CAD build for the part. Positions are in the model's coordinates, mm. A direction names the side the tool comes from. Give positions to 0.01 mm unless a question says otherwise; leave off trailing zeros. Order: outer loops, then holes, each group sorted by start corner. A loop starts at its lowest first (then second) coordinate and runs counter-clockwise, first axis right, second up.
from build123d import *

# Parameters (mm, degrees)
F0_R     = 16.5
F1_DEPTH = 30
F2_W     = 12.5
F2_H     = 30
F3_DEPTH = 17
F4_R     = 9.5
F5_DEPTH = 15
F6_R     = 10.5
F7_DEPTH = 15
F8_R     = 5
F9_DEPTH = 77


with BuildPart() as f1:
    # F0 (on Front) → F1 (new body)
    with BuildSketch(Plane.XZ):
        Circle(F0_R)
    extrude(amount=F1_DEPTH)

    # F2 (on Top) → F3 (join)
    with BuildSketch(Plane.XY):
        with Locations((6.25, -15)):
            Rectangle(F2_W, F2_H)
        with Locations((-6.25, -15)):
            Rectangle(F2_W, F2_H)
    extrude(amount=F3_DEPTH)

    # F4 (on face) → F5 (join)
    with BuildSketch(Plane.XZ.offset(30)):
        Circle(F4_R)
    extrude(amount=F5_DEPTH)

    # F6 (on Front) → F7 (cut)
    with BuildSketch(Plane.XZ):
        Circle(F6_R)
    extrude(amount=F7_DEPTH, mode=Mode.SUBTRACT)

    # F8 (on face) → F9 (cut)
    with BuildSketch(Plane.XZ.offset(45)):
        Circle(F8_R)
    extrude(amount=-F9_DEPTH, mode=Mode.SUBTRACT)


solid = f1.part
1. 3-axis set-ups, long thin cutter, end or side, ignore diameter. For faces 5 (the flat face through (-8, 0, 8)), 6 (the flat face through (5, -15, -2)), 7 (the cylindrical face through (-1.08, -30.21, -4.88)), 8 (the cylindrical face through (4.38, -37.39, -8.43)), 9 (the flat face through (12.5, -15, 14)): which of +Z, -Z, +X, -X, +Y, -Y reach the whole face in a straight line?
2. Wall check: line 1 (Z direction, x = 0, y = -35); line 2 (Z direction, x = 0, y = -19.5); line 3 (Y direction, x = 15, z = 0.5). Give the ranges that are in metal, low to high.
3. Saw through at D-D on z = 15. Give the cut face in (x, y).
4. Saw through at B-B on x = 0. Give the cut face in (y, z).
5. Saw through at C-C on y = -3. Give the cut face in (x, z), plus the area to 3 significant figures.
6. Mould opens along X. For faces 1 (the flat face through (4, -45, -4)), 2 (the cylindrical face through (-0.53, -14.79, -16.49)), 3 (the flat face through (-12.5, -15, 14)), 4 (the cylindrical face through (10, -7.4, 3.2)) say: released by +X, released by -X, zero draft, split by the parting line, or undercut.
7. Pin check, flat tips, straight feed: P1, Ø10, axis at x = -10.5, y = -23, coming from the -Z side; P2, Ø17, axis at x = -1, z = -0.5, coming from the +Y side; P3, Ø5, axis at y = -16.5, z = 14, coming from the +X side. Stop position of each tip, or through.
8. Saw through at A-A on z = 0. Give the cut face in (x, y), plus the area to 3 significant figures.
Reported:
1. face 5: +Z, -Z, +X, -X, +Y
1. face 6: +Y
1. face 7: +Y, -Y
1. face 8: -Y
1. face 9: +Z, +X, +Y, -Y
2. line 1: z = -9.5 to -5, 5 to 9.5
2. line 2: z = -16.5 to -5, 5 to 17
2. line 3: y = -30 to 0
3. outline: (-12.5, -30) - (12.5, -30) - (12.5, 0) - (-12.5, 0) - close
4. outline: (-45, -9.5) - (-30, -9.5) - (-30, -16.5) - (0, -16.5) - (0, -10.5) - (-15, -10.5) - (-15, -5) - (-45, -5) - close; (-45, 5) - (-15, 5) - (-15, 10.5) - (0, 10.5) - (0, 17) - (-30, 17) - (-30, 9.5) - (-45, 9.5) - close
5. outline: (-12.5, 10.77) arc R16.5 ccw (long way) to (12.5, 10.77) - (12.5, 17) - (-12.5, 17) - close; hole circle Ø21 at (0, 0)
5. area: 565 mm2
6. face 1: zero draft
6. face 2: split by the parting line
6. face 3: released by -X
6. face 4: undercut
7. P1: stops at z = -15.56
7. P2: stops at y = -15
7. P3: stops at x = 12.5
8. outline: (-16.5, -30) - (-9.5, -30) - (-9.5, -45) - (-5, -45) - (-5, -15) - (-10.5, -15) - (-10.5, 0) - (-16.5, 0) - close; (5, -45) - (9.5, -45) - (9.5, -30) - (16.5, -30) - (16.5, 0) - (10.5, 0) - (10.5, -15) - (5, -15) - close
8. area: 660 mm2
